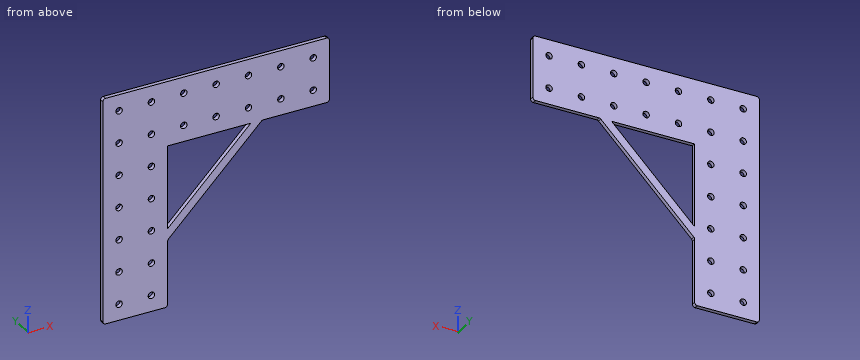
from build123d import *

# Parameters (mm, degrees)
SKETCH1_R           = 2.54
BOSS_EXTRUDE1_DEPTH = 3.175


with BuildPart() as part:
    # Sketch1 → Boss-Extrude1 (new body)
    with BuildSketch(Plane(origin=(0, 0, 0), x_dir=(1, 0, 0), z_dir=(0, 1, 0))):
        with BuildLine():
            Line((-92.728830313, 61.050098366), (-92.728830313, -112.561465747))
            ThreePointArc((-92.728830313, -112.561465747), (-92.115448079, -114.042301456), (-90.63461237, -114.65568369))
            Line((-90.63461237, -114.65568369), (82.976951744, -114.65568369))
            ThreePointArc((82.976951744, -114.65568369), (84.457787453, -114.042301456), (85.071169687, -112.561465747))
            Line((85.071169687, -112.561465747), (85.071169687, -65.949901634))
            ThreePointArc((85.071169687, -65.949901634), (84.457787453, -64.469065925), (82.976951744, -63.85568369))
            Line((82.976951744, -63.85568369), (33.202051993, -63.85568369))
            ThreePointArc((33.202051993, -63.85568369), (32.400629482, -63.696270841), (31.721216284, -63.242301456))
            Line((31.721216284, -63.242301456), (-41.315448079, 9.794362906))
            ThreePointArc((-41.315448079, 9.794362906), (-41.769417464, 10.473776105), (-41.928830313, 11.275198615))
            Line((-41.928830313, 11.275198615), (-41.928830313, 61.050098366))
            ThreePointArc((-41.928830313, 61.050098366), (-42.542212547, 62.530934075), (-44.023048256, 63.14431631))
            Line((-44.023048256, 63.14431631), (-90.63461237, 63.14431631))
            ThreePointArc((-90.63461237, 63.14431631), (-92.115448079, 62.530934075), (-92.728830313, 61.050098366))
        make_face()
        with Locations(Location((-80.028830313, 50.44431631, 0), (0, 0, 270))):
            Circle(SKETCH1_R, mode=Mode.SUBTRACT)
        with Locations(Location((-54.628830313, 50.44431631, 0), (0, 0, 270))):
            Circle(SKETCH1_R, mode=Mode.SUBTRACT)
        with Locations(Location((-54.628830313, 25.04431631, 0), (0, 0, 270))):
            Circle(SKETCH1_R, mode=Mode.SUBTRACT)
        with Locations(Location((-54.628830313, -0.35568369, 0), (0, 0, 270))):
            Circle(SKETCH1_R, mode=Mode.SUBTRACT)
        with Locations(Location((-54.628830313, -25.75568369, 0), (0, 0, 270))):
            Circle(SKETCH1_R, mode=Mode.SUBTRACT)
        with Locations(Location((-54.628830313, -51.15568369, 0), (0, 0, 270))):
            Circle(SKETCH1_R, mode=Mode.SUBTRACT)
        with Locations(Location((-80.028830313, 25.04431631, 0), (0, 0, 270))):
            Circle(SKETCH1_R, mode=Mode.SUBTRACT)
        with Locations(Location((-80.028830313, -0.35568369, 0), (0, 0, 270))):
            Circle(SKETCH1_R, mode=Mode.SUBTRACT)
        with Locations(Location((-80.028830313, -25.75568369, 0), (0, 0, 270))):
            Circle(SKETCH1_R, mode=Mode.SUBTRACT)
        with Locations(Location((-80.028830313, -51.15568369, 0), (0, 0, 270))):
            Circle(SKETCH1_R, mode=Mode.SUBTRACT)
        with Locations(Location((-80.028830313, -76.55568369, 0), (0, 0, 270))):
            Circle(SKETCH1_R, mode=Mode.SUBTRACT)
        with Locations(Location((-54.628830313, -76.55568369, 0), (0, 0, 270))):
            Circle(SKETCH1_R, mode=Mode.SUBTRACT)
        with Locations(Location((-80.028830313, -101.95568369, 0), (0, 0, 270))):
            Circle(SKETCH1_R, mode=Mode.SUBTRACT)
        with Locations(Location((-54.628830313, -101.95568369, 0), (0, 0, 270))):
            Circle(SKETCH1_R, mode=Mode.SUBTRACT)
        with Locations(Location((-29.228830313, -101.95568369, 0), (0, 0, 270))):
            Circle(SKETCH1_R, mode=Mode.SUBTRACT)
        with Locations(Location((-3.828830313, -101.95568369, 0), (0, 0, 270))):
            Circle(SKETCH1_R, mode=Mode.SUBTRACT)
        with Locations(Location((21.571169687, -101.95568369, 0), (0, 0, 270))):
            Circle(SKETCH1_R, mode=Mode.SUBTRACT)
        with Locations(Location((46.971169687, -101.95568369, 0), (0, 0, 270))):
            Circle(SKETCH1_R, mode=Mode.SUBTRACT)
        with Locations(Location((72.371169687, -101.95568369, 0), (0, 0, 270))):
            Circle(SKETCH1_R, mode=Mode.SUBTRACT)
        with Locations(Location((-3.828830313, -76.55568369, 0), (0, 0, 270))):
            Circle(SKETCH1_R, mode=Mode.SUBTRACT)
        with Locations(Location((21.571169687, -76.55568369, 0), (0, 0, 270))):
            Circle(SKETCH1_R, mode=Mode.SUBTRACT)
        with Locations(Location((46.971169687, -76.55568369, 0), (0, 0, 270))):
            Circle(SKETCH1_R, mode=Mode.SUBTRACT)
        with Locations(Location((72.371169687, -76.55568369, 0), (0, 0, 270))):
            Circle(SKETCH1_R, mode=Mode.SUBTRACT)
        with Locations(Location((-29.228830313, -76.55568369, 0), (0, 0, 270))):
            Circle(SKETCH1_R, mode=Mode.SUBTRACT)
        Polygon((-41.928830313, 1.42748902), (-41.928830313, -63.85568369), (23.354342397, -63.85568369), align=None, mode=Mode.SUBTRACT)
    extrude(amount=BOSS_EXTRUDE1_DEPTH)


solid = part.part
Can you work these out from the model? Positions are in its coordinate system, mm. Round coordinates to 2 decimals unless told otherwise and drop trailing zeros. Write each loop counter-clockwise with the first axis right and the second up, starting at its lowest first coordinate (ties: lowest second). Pieces come first, ordered by that corner, then holes. Notation, with made-up numbers: M 5,23 L 14,23 A12 ccw 14,34 Z; hole C 1,43.5 d7. An arc over 180 degrees is marked long. Use CSV: the item, a comma, the result in double quotes.
(1) I need wall thicknesses on line 1 along Z through (x, y) = (-30, 0.2); line 2 along Z through (x, y) = (72.5, 2); line 3 along X through (y, z) = (1.3, -0.5). Which ranges of each line are inside material? Lowest first, please.
Check values:
line 1,"1.52 to 10.5, 63.86 to 74.14, 78.98 to 99.54, 104.38 to 114.66"
line 2,"63.86 to 74.02, 79.09 to 99.42, 104.49 to 114.66"
line 3,"-92.73 to -82.42, -77.64 to -57.02, -52.24 to -41.93, -41 to -32.02"
(2) Imagine slicing it at A-A (x = -10.5). Write out the boundary of the cut face in (y, z) (3 decimals), plus the area to 3 significant figures.
Check values:
outline,"M 0,21.021 L 3.175,21.021 L 3.175,30.001 L 0,30.001 Z; M 0,63.856 L 3.175,63.856 L 3.175,114.656 L 0,114.656 Z"
area,"190 mm^2"
(3) Imagine slicing it at B-B (y = 2.65). Count the separate pieces of the cut face and the enclosed holes in it, plus the area to 3 significant figures.
Check values:
separate pieces,"1"
enclosed holes,"25"
area,"15,600 mm^2"
